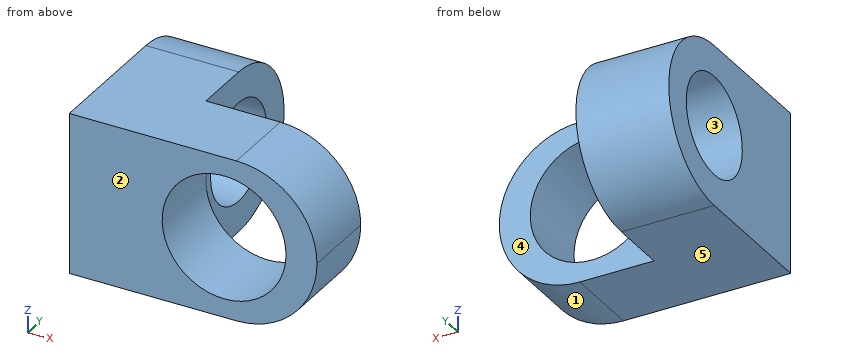
```python
from build123d import *

# Parameters (mm, degrees)
SKETCH1_R           = 1.6
BOSS_EXTRUDE1_DEPTH = 3
SKETCH2_W           = 5.2
SKETCH2_H           = 2.5
BOSS_EXTRUDE2_DEPTH = 5
FILLET1_R           = 2.6
SKETCH3_R           = 2
CUT_EXTRUDE1_DEPTH  = 5


with BuildPart() as part:
    # Sketch1 → Boss-Extrude1 (new body)
    with BuildSketch(Plane(origin=(0, 0, 0), x_dir=(0, 0, -1), z_dir=(1, 0, 0))):
        with BuildLine():
            ThreePointArc((2.6, 0), (0, 2.6), (-2.6, 0))
            Line((-2.6, 0), (-2.6, -4.365701483))
            Line((-2.6, -4.365701483), (2.6, -4.365701483))
            Line((2.6, -4.365701483), (2.6, 0))
        make_face()
        Circle(SKETCH1_R, mode=Mode.SUBTRACT)
    extrude(amount=BOSS_EXTRUDE1_DEPTH)

    # Sketch2 → Boss-Extrude2 (add)
    with BuildSketch(Plane(origin=(3, 0, 0), x_dir=(0, 0, -1), z_dir=(1, 0, 0))):
        with Locations((0, -3.115701483)):
            Rectangle(SKETCH2_W, SKETCH2_H)
    extrude(amount=BOSS_EXTRUDE2_DEPTH)

    # Fillet1
    fillet1_edges = [part.edges().sort_by_distance(p)[0] for p in [
        (8, -3.115701483, -2.6),
        (8, -3.115701483, 2.6),
    ]]
    fillet(fillet1_edges, radius=FILLET1_R - 0.0001)  # a hair under: the kernel refuses the full size

    # Sketch3 → Cut-Extrude1 (cut)
    with BuildSketch(Plane.XZ.offset(4.365701483)):
        with Locations(Location((5, 0, 0), (0, 0, 270))):
            Circle(SKETCH3_R)
    extrude(amount=-CUT_EXTRUDE1_DEPTH, mode=Mode.SUBTRACT)


solid = part.part
```
Geometry check sheet. Reference: the model listing, model coordinates, mm. Face numbers are marked on the shaded views. A direction names the side the tool comes from. Round coordinates to 2 decimals unless told otherwise and drop trailing zeros. Order: outer loops, then holes, each group sorted by start corner. A loop starts at its lowest first (then second) coordinate and runs counter-clockwise, first axis right, second up. Notation, with made-up numbers: M 81,78 L 119,78 A31 cw 119,117 Z; hole C 38,59.5 d6. An arc over 180 degrees is marked long. Write item = value, one per line.
Q1. Depth check by flat-ended pin: pin 1 Ø1.5 at (x, z) = (6, 0.5) entering from +Y; pin 2 Ø1.5 at (y, z) = (-1, 1) entering from +X. Enter the tip coordinate at first touch or a pass-through.
Answer block:
pin_1 = through
pin_2 = 3
Q2. Scan lines: line 1 (X direction, y = -2.55, z = 0); line 2 (Y direction, x = 1.35, z = 0); line 3 (Z direction, x = 5, y = -3.5). Record each from-to range of solid material in increasing order.
Answer block:
line_1 = 0 to 3, 7 to 8
line_2 = -4.37 to -1.6, 1.6 to 2.6
line_3 = -2.6 to -2, 2 to 2.6
Q3. Section check D-D (z = 0.45). Enter the section's corners in (x, y).
Answer block:
outline = M 0,-4.37 L 3.05,-4.37 L 3.05,-1.87 L 3,-1.87 L 3,-1.54 L 0,-1.54 Z; M 0,1.54 L 3,1.54 L 3,2.56 L 0,2.56 Z; M 6.95,-4.37 L 7.96,-4.37 L 7.96,-1.87 L 6.95,-1.87 Z
Q4. Section check C-C (y = 0.5). Enter the section's corners in (x, z), plus the area to 3 significant figures.
Answer block:
outline = M 0,-2.55 L 3,-2.55 L 3,-1.52 L 0,-1.52 Z; M 0,1.52 L 3,1.52 L 3,2.55 L 0,2.55 Z
area = 6.19 mm^2
Q5. Section check B-B (x = 5). Enter the section's corners in (y, z), plus the area to 3 significant figures.
Answer block:
outline = M -4.37,-2.6 L -1.87,-2.6 L -1.87,-2 L -4.37,-2 Z; M -4.37,2 L -1.87,2 L -1.87,2.6 L -4.37,2.6 Z
area = 3.00 mm^2
Q6. Release check for a two-part mould opening along Y. For the marked faces 1, 2 and 3 record: released by +Y, released by -Y, zero draft, split by the parting line, or undercut.
Answer block:
face_1 = zero draft
face_2 = released by -Y
face_3 = undercut
Q7. Set-up check for the marked faces 4 and 5: record each of +Z, -Z, +X, -X, +Y, -Y from which the full face is reachable in a straight line by a thin tool's end or side.
Answer block:
face_4 = +Z, -Z, +X, +Y
face_5 = -Z, +X, -X, +Y, -Y
